from build123d import *

# Parameters (mm, degrees)
SM_BASE_FLANGE_1_DEPTH       = 50
HOLE_WIZARD_1_AT_2_COUNT     = 2
HOLE_WIZARD_1_AT_2_PITCH     = 37.643060449
HOLE_WIZARD_1_AT_3_COUNT     = 2
HOLE_WIZARD_1_AT_3_PITCH     = 37.643060449
HOLE_WIZARD_4_2_4_2_1_D      = 4.2
HOLE_WIZARD_4_2_4_2_2_REACH  = 232.331
HOLE_WIZARD_4_2_4_2_2_BORE_R = 2.1
CUT_EXTRUDE_1_DEPTH          = 134.839456066
HOLE_WIZARD_5_0_5_1_D        = 5


# Read off the part's stored shape, not the designer's step: 基体-法兰1
with BuildPart() as part:
    # 基体-法兰1 outline → 基体-法兰1 (new body)
    with BuildSketch(Plane.XY):
        with BuildLine():
            Line((102.5, 0), (122, 0))
            Line((122, 0), (122, 1.5))
            Line((122, 1.5), (102.5, 1.5))
            ThreePointArc((102.5, 1.5), (101.792893219, 1.792893219), (101.5, 2.5))
            Line((101.5, 2.5), (101.5, 22))
            ThreePointArc((101.5, 22), (100.767766953, 23.767766953), (99, 24.5))
            Line((99, 24.5), (-99, 24.5))
            ThreePointArc((-99, 24.5), (-100.767766953, 23.767766953), (-101.5, 22))
            Line((-101.5, 22), (-101.5, 2.5))
            ThreePointArc((-101.5, 2.5), (-101.792893219, 1.792893219), (-102.5, 1.5))
            Line((-102.5, 1.5), (-122, 1.5))
            Line((-122, 1.5), (-122, 0))
            Line((-122, 0), (-102.5, 0))
            ThreePointArc((-102.5, 0), (-100.732233047, 0.732233047), (-100, 2.5))
            Line((-100, 2.5), (-100, 22))
            ThreePointArc((-100, 22), (-99.707106781, 22.707106781), (-99, 23))
            Line((-99, 23), (99, 23))
            ThreePointArc((99, 23), (99.707106781, 22.707106781), (100, 22))
            Line((100, 22), (100, 2.5))
            ThreePointArc((100, 2.5), (100.732233047, 0.732233047), (102.5, 0))
        make_face()
    extrude(amount=SM_BASE_FLANGE_1_DEPTH)

    # 草图9 → 打孔尺寸(%根据)开槽沉头木螺钉的类型1 (revolve, cut)
    with BuildSketch(Plane(origin=(0, 24.5, 4), x_dir=(0, 0, 1), z_dir=(1, 0, 0))):
        Polygon((0, 0), (0, 1.5), (1.7, 1.5), (1.7, 1.6), (3.3, 0), align=None)
    hole_wizard_1 = revolve(axis=Axis((0, 30.85, 4), (0, -1, 0)), mode=Mode.SUBTRACT)

    # 打孔尺寸(%根据)开槽沉头木螺钉的类型1 at 2: 打孔尺寸(%根据)开槽沉头木螺钉的类型1 ×2
    with Locations(*[Vector(-0.29221853559902017, 0, 0.956351571051339) * (i * HOLE_WIZARD_1_AT_2_PITCH) for i in range(1, HOLE_WIZARD_1_AT_2_COUNT)]):
        add(hole_wizard_1, mode=Mode.SUBTRACT)

    # 打孔尺寸(%根据)开槽沉头木螺钉的类型1 at 3: 打孔尺寸(%根据)开槽沉头木螺钉的类型1 ×2
    with Locations(*[Vector(0.2922185355990204, 0, 0.956351571051339) * (i * HOLE_WIZARD_1_AT_3_PITCH) for i in range(1, HOLE_WIZARD_1_AT_3_COUNT)]):
        add(hole_wizard_1, mode=Mode.SUBTRACT)

    # Ø4.2 (4.2) 直径孔1 (through all)
    with Locations(Plane(origin=(0, 24.5, 0), x_dir=(1, 0, 0), z_dir=(0, 1, 0))):
        with Locations((-40, -42), (-80, -42), (40, -42), (80, -42)):
            Hole(HOLE_WIZARD_4_2_4_2_1_D / 2)

    # Ø4.2 (4.2) 直径孔2 bore → Ø4.2 (4.2) 直径孔2 (cut, up to next)
    with BuildSketch(Plane(origin=(101.5, 0, 0), x_dir=(0, 0, -1), z_dir=(1, 0, 0)), mode=Mode.PRIVATE) as hole_wizard_4_2_4_2_2_sk1:
        with Locations((-42, 6.5)):
            Circle(HOLE_WIZARD_4_2_4_2_2_BORE_R)
    hole_wizard_4_2_4_2_2_tool1 = extrude(hole_wizard_4_2_4_2_2_sk1.sketch, amount=-HOLE_WIZARD_4_2_4_2_2_REACH, mode=Mode.PRIVATE) & part.part
    hole_wizard_4_2_4_2_2 = hole_wizard_4_2_4_2_2_tool1.solids().sort_by_distance((101.5, 6.5, 42))[0]
    add(hole_wizard_4_2_4_2_2, mode=Mode.SUBTRACT)

    # 镜向1: Ø4.2 (4.2) 直径孔2 across plane
    add(hole_wizard_4_2_4_2_2.mirror(Plane(origin=(0, 0, 0), x_dir=(0, 0, 1), z_dir=(1, 0, 0))), mode=Mode.SUBTRACT)

    # 草图15 → 切除-拉伸1 (cut, through all)
    with BuildSketch(Plane(origin=(0, 1.5, 0), x_dir=(1, 0, 0), z_dir=(0, 1, 0))):
        with BuildLine():
            Line((-117, -2.9), (-107, -2.9))
            ThreePointArc((-107, -2.9), (-104.9, -5), (-107, -7.1))
            Line((-107, -7.1), (-117, -7.1))
            ThreePointArc((-117, -7.1), (-119.1, -5), (-117, -2.9))
        make_face()
        with BuildLine():
            Line((-117, -42.9), (-107, -42.9))
            ThreePointArc((-107, -42.9), (-104.9, -45), (-107, -47.1))
            Line((-107, -47.1), (-117, -47.1))
            ThreePointArc((-117, -47.1), (-119.1, -45), (-117, -42.9))
        make_face()
    cut_extrude_1 = extrude(amount=-CUT_EXTRUDE_1_DEPTH, mode=Mode.SUBTRACT)

    # 镜向2: 切除-拉伸1 across plane
    add(cut_extrude_1.mirror(Plane(origin=(0, 0, 0), x_dir=(0, 0, 1), z_dir=(1, 0, 0))), mode=Mode.SUBTRACT)

    # Ø5.0 (5) 直径孔1 (through all)
    with Locations(Plane(origin=(0, 24.5, 0), x_dir=(1, 0, 0), z_dir=(0, 1, 0))):
        with Locations((-8, -31)):
            Hole(HOLE_WIZARD_5_0_5_1_D / 2)


solid = part.part
Can you work these out from the model? Positions are in its coordinate system, mm. A direction names the side the tool comes from. Round coordinates to 2 decimals unless told otherwise and drop trailing zeros. Loops run counter-clockwise (first coordinate to the right, second up) from the corner with the lowest first, then second, coordinate; pieces in that order, holes last. Notation, with made-up numbers: (21.25, 13.25) - (26.25, 13.25) arc R24 ccw to (26.25, 49.25) - close; hole circle Ø3 at (-31, 65.25). An arc over 180 degrees is marked (long way). Answer in a Markdown table with one row per item. Add a question column.
Q1. I want a section at B-B on x = 11. List the corners of the cut face in (y, z) for me, and give its area (4 significant figures).
Q2. I want a section at D-D on z = 16. List the corners of the cut face in (x, y) for me.
Q3. We'd pull the mould along Y, two halves only. Please class faces 1 (the flat face through (-0.6, 23.2, 50)), 2 (the cylindrical face through (100.76, 8.582, 42.273)), 3 (the flat face through (112, 1.5, 25)): pulls with the +Y half, pulls with the -Y half, needs draft (parallel to the pull), parting line crosses it, or undercut.
Q4. For pin 1 Ø10 at (x, z) = (-111, 33.5) entering from +Y; pin 2 Ø6 at (y, z) = (16.5, 42) entering from +X; pin 3 Ø4 at (x, z) = (-84.5, 9.5) entering from -Y; pin 4 Ø2.5 at (y, z) = (6.5, 42) entering from -X, each with a flat end and sliding along its axis, tell me the tip position at first contact or that it passes through.
Q5. I need wall thicknesses on L1, parallel to X at y = 9.5, z = 14.5; L2, parallel to Z at x = 80, y = 23.55; L3, parallel to Y at x = 31, z = 12. Which ranges of each line are inside material? Lowest first, please.
Q6. I want a section at A-A on y = 17.5. List the corners of the cut face in (x, z) for me, and give its area (3 significant figures).
Q7. Which directions (+Z, -Z, +X, -X, +Y, -Y) give clear straight access to the entire face, cutting with the end or side of a thin tool? Please do faces 4 (the cylindrical face through (-9.34, 23.74, 28.89)), 5 (the flat face through (101.5, 12, 25)), 6 (the flat face through (-101.5, 12, 25)), 7 (the flat face through (-100, 12, 25)).
Q8. I want a section at C-C on y = 6.5. List the corners of the cut face in (x, z) for me, and give its area (3 significant figures).
A:
| question | item | result |
|---|---|---|
| 1 | outline | (23, 0) - (24.5, 0) - (24.5, 36.7) - (23, 38.2) - close; (23, 41.8) - (24.5, 43.3) - (24.5, 50) - (23, 50) - close |
| 1 | area | 67.35 mm^2 |
| 2 | outline | (-122, 0) - (-102.5, 0) arc R2.5 ccw to (-100, 2.5) - (-100, 22) arc R1 cw to (-99, 23) - (99, 23) arc R1 cw to (100, 22) - (100, 2.5) arc R2.5 ccw to (102.5, 0) - (122, 0) - (122, 1.5) - (102.5, 1.5) arc R1 cw to (101.5, 2.5) - (101.5, 22) arc R2.5 ccw to (99, 24.5) - (-99, 24.5) arc R2.5 ccw to (-101.5, 22) - (-101.5, 2.5) arc R1 cw to (-102.5, 1.5) - (-122, 1.5) - close |
| 3 | face 1 | needs draft |
| 3 | face 2 | undercut |
| 3 | face 3 | pulls with the +Y half |
| 4 | pin 1 | y = 1.5 |
| 4 | pin 2 | x = 101.5 |
| 4 | pin 3 | y = 23 |
| 4 | pin 4 | through |
| 5 | L1 | -101.5 to -100, 100 to 101.5 |
| 5 | L2 | 0 to 39.9, 44.1 to 50 |
| 5 | L3 | 23 to 24.5 |
| 6 | outline | (-101.5, 0) - (-100, 0) - (-100, 50) - (-101.5, 50) - close; (100, 0) - (101.5, 0) - (101.5, 50) - (100, 50) - close |
| 6 | area | 150 mm^2 |
| 7 | face 4 | +Y, -Y |
| 7 | face 5 | +Z, -Z, +X, +Y |
| 7 | face 6 | +Z, -Z, -X, +Y |
| 7 | face 7 | +Z, -Z, -Y |
| 8 | outline | (-101.5, 0) - (-100, 0) - (-100, 39.9) - (-101.5, 39.9) - close; (-101.5, 44.1) - (-100, 44.1) - (-100, 50) - (-101.5, 50) - close; (100, 0) - (101.5, 0) - (101.5, 39.9) - (100, 39.9) - close; (100, 44.1) - (101.5, 44.1) - (101.5, 50) - (100, 50) - close |
| 8 | area | 137 mm^2 |
